from build123d import *

# Parameters (mm, degrees)
SCHIZZO1_W                   = 10
SCHIZZO1_H                   = 5
ESTRUSIONE_ESTRUSIONE1_DEPTH = 15
SCHIZZO2_R                   = 1.5
TAGLIO_ESTRUSIONE1_DEPTH     = 19.708286934


with BuildPart() as part:
    # Schizzo1 → Estrusione-Estrusione1 (new body)
    with BuildSketch(Plane.XY):
        with Locations((-5, 2.5)):
            Rectangle(SCHIZZO1_W, SCHIZZO1_H)
    extrude(amount=ESTRUSIONE_ESTRUSIONE1_DEPTH)

    # Schizzo2 → Taglio-Estrusione1 (cut, through all)
    with BuildSketch(Plane(origin=(0, 0, 0), x_dir=(-1, 0, 0), z_dir=(0, -1, 0))):
        with Locations(Location((5, -12, 0), (0, 0, 180))):
            Circle(SCHIZZO2_R)
        with Locations(Location((5, -3, 0), (0, 0, 180))):
            Circle(SCHIZZO2_R)
    extrude(amount=-TAGLIO_ESTRUSIONE1_DEPTH, mode=Mode.SUBTRACT)


solid = part.part
Input: part model. Units: mm. Frame: model coordinates. Give positions to 0.01 mm unless a question says otherwise; leave off trailing zeros. Loops run counter-clockwise (first coordinate to the right, second up) from the corner with the lowest first, then second, coordinate; pieces in that order, holes last. Notation, with made-up numbers: (14, 6) -> (37, 6) arc R18 cw to (37, 39) -> close; hole circle Ø5 at (37.5, 34.5). An arc over 180 degrees is marked (long way). Answer as a JSON object with one key per item and string values. Group by question number.
Item 1: Line query: probe 1 along Z at (x, y) = (-5, 2.95); probe 2 along Z at (x, y) = (-5.75, 2.1); probe 3 along X at (y, z) = (0.75, 4). Output: solid intervals per line, ascending.
Item 2: Cut plane A-A, the plane z = 12. Return the cut outline in (x, y), and give its area (3 significant figures).
Item 3: Cut plane C-C, the plane y = 0.9. Return the cut outline in (x, z), and give its area (3 significant figures).
Item 4: Pull-direction query (Z, two-part tool) for faces 1 (the cylindrical face through (-6.2, 2.5, 2.1)), 2 (the flat face through (-5, 3, 0)), 3 (the flat face through (-5, 0, 7)); classes: released by +Z, released by -Z, zero draft, split by the parting line, or undercut.
Item 5: Cut plane D-D, the plane z = 4. Return the cut outline in (x, y), and give its area (3 significant figures).
Item 6: Pin query (flat end, axial travel): P1, Ø3, axis at y = 4, z = 9, coming from the +X side. Return the tip coordinate at first contact, or that it passes through.
Item 7: Cut plane B-B, the plane x = -5. Return the cut outline in (y, z).
Checks:
{
 "1": {"probe 1": "z = 0 to 1.5, 4.5 to 10.5, 13.5 to 15", "probe 2": "z = 0 to 1.7, 4.3 to 10.7, 13.3 to 15", "probe 3": "x = -10 to -6.12, -3.88 to 0"},
 "2": {"outline": "(-10, 0) -> (-6.5, 0) -> (-6.5, 5) -> (-10, 5) -> close; (-3.5, 0) -> (0, 0) -> (0, 5) -> (-3.5, 5) -> close", "area": "35.0 mm²"},
 "3": {"outline": "(-10, 0) -> (0, 0) -> (0, 15) -> (-10, 15) -> close; hole circle Ø3 at (-5, 3); hole circle Ø3 at (-5, 12)", "area": "136 mm²"},
 "4": {"face 1": "undercut", "face 2": "released by -Z", "face 3": "zero draft"},
 "5": {"outline": "(-10, 0) -> (-6.12, 0) -> (-6.12, 5) -> (-10, 5) -> close; (-3.88, 0) -> (0, 0) -> (0, 5) -> (-3.88, 5) -> close", "area": "38.8 mm²"},
 "6": {"P1": "stops at x = 0"},
 "7": {"outline": "(0, 0) -> (5, 0) -> (5, 1.5) -> (0, 1.5) -> close; (0, 4.5) -> (5, 4.5) -> (5, 10.5) -> (0, 10.5) -> close; (0, 13.5) -> (5, 13.5) -> (5, 15) -> (0, 15) -> close"}
}
